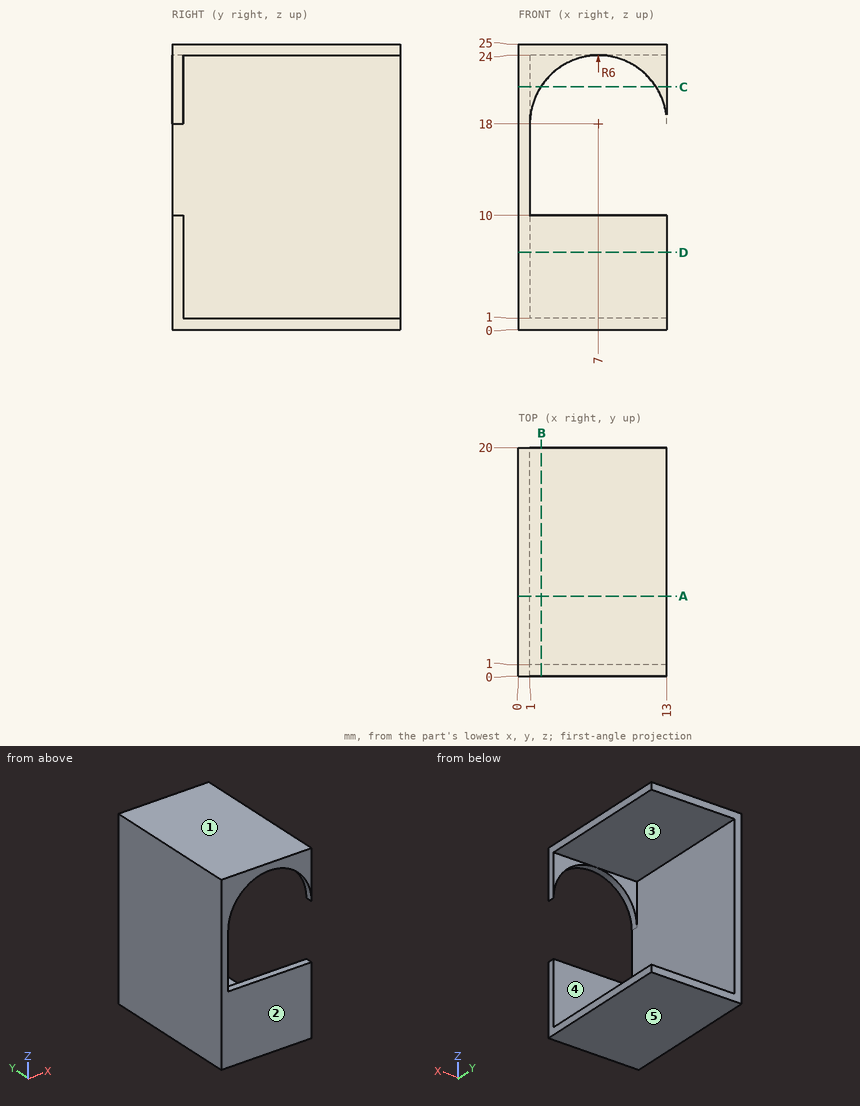
Print and shaded views of the part. All mm, measured from the part's lowest x, y and z. A direction names the side the tool comes from. Coordinates: 2 decimals unless noted, no trailing zeros. Order: outer loops, then holes, each group sorted by start corner. A loop starts at its lowest first (then second) coordinate and runs counter-clockwise, first axis right, second up. Notation, with made-up numbers: (45.5, 71.5) - (100.5, 71.5) arc R16 ccw to (100.5, 102.5) - close; hole circle Ø4 at (53.25, 15.25). An arc over 180 degrees is marked (long way). Return JSON: item names as keys, results as strings. Group by question number.
Item 1: Cut at A-A (y = 7). List the corners of the cut face in (x, z).
Item 2: Drill centre lines: probe 1 along Z at (x, y) = (4.5, 9.5); probe 2 along Y at (x, z) = (10.5, 2.25). Where is each one in solid material? Low to high. Write a range as from..to.
Item 3: Pin check, flat tips, straight feed: pin 1 (6 mm diameter, centred on y = 12.5, z = 14.5, fed in from +X); pin 2 (5 mm diameter, centred on x = 5, z = 20, fed in from +Y); pin 3 (5 mm diameter, centred on x = 10.5, z = 19.5, fed in from +Y). Stop position of each tip, or through.
Item 4: Which spindle directions (+Z, -Z, +X, -X, +Y, -Y) get a long thin tool onto all of the face, cutting with end or side? Do the marked faces 4 and 5. Say none if no direction does.
Item 5: Cut at B-B (x = 2). List the corners of the cut face in (y, z).
Item 6: Pull direction Z, two halves, no side cores. Call the marked faces 1, 2 and 3: pulls with the +Z half, pulls with the -Z half, needs draft (parallel to the pull), parting line crosses it, or undercut.
Item 7: Cut at D-D (z = 6.75). List the corners of the cut face in (x, y), plus the area to 3 significant figures.
Item 8: Cut at C-C (z = 21.25). List the corners of the cut face in (x, y).
Check values:
{
 "1": {"outline": "(0, 0) - (13, 0) - (13, 1) - (1, 1) - (1, 24) - (13, 24) - (13, 25) - (0, 25) - close"},
 "2": {"probe 1": "z = 0..1, 24..25", "probe 2": "y = 0..1"},
 "3": {"pin 1": "stops at x = 1", "pin 2": "passes through", "pin 3": "stops at y = 1"},
 "4": {"face 4": "+X, +Y", "face 5": "-Z, +X, -X, +Y, -Y"},
 "5": {"outline": "(0, 0) - (20, 0) - (20, 1) - (1, 1) - (1, 10) - (0, 10) - close; (0, 21.32) - (1, 21.32) - (1, 24) - (20, 24) - (20, 25) - (0, 25) - close"},
 "6": {"face 1": "pulls with the +Z half", "face 2": "needs draft", "face 3": "undercut"},
 "7": {"outline": "(0, 0) - (13, 0) - (13, 1) - (1, 1) - (1, 20) - (0, 20) - close", "area": "32.0 mm2"},
 "8": {"outline": "(0, 0) - (1.96, 0) - (1.96, 1) - (1, 1) - (1, 20) - (0, 20) - close; (12.04, 0) - (13, 0) - (13, 1) - (12.04, 1) - close"}
}
